Verification items for the finished model (mm, model axes). A direction names the side the tool comes from. Give positions to 0.01 mm unless a question says otherwise; leave off trailing zeros. Loops run counter-clockwise (first coordinate to the right, second up) from the corner with the lowest first, then second, coordinate; pieces in that order, holes last. Notation, with made-up numbers: (-6.75, 66) -> (10.25, 66) arc R21 ccw to (10.25, 74) -> close; hole circle Ø9 at (1.25, 38). An arc over 180 degrees is marked (long way). Use one line per item in the form item = value. Start each with the question number.
from build123d import *

# Parameters (mm, degrees)
BOARD_DEPTH        = 1.68
SKETCH2_R          = 0.2032
SKETCH2_R_2        = 0.4699
SKETCH2_R_3        = 1.5875
SKETCH2_R_4        = 0.4953
PLATED_HOLES_DEPTH = 2.68


with BuildPart() as part:
    # Sketch1 → BOARD (new body)
    with BuildSketch(Plane.XY):
        with BuildLine():
            Line((60, 63), (60, 61))
            ThreePointArc((60, 61), (60.585786438, 59.585786438), (62, 59))
            Line((62, 59), (77.171572667, 59))
            ThreePointArc((77.171572667, 59), (77.936939773, 58.847758994), (78.585786667, 58.414213333))
            Line((78.585786667, 58.414213333), (84.414213333, 52.585786667))
            ThreePointArc((84.414213333, 52.585786667), (85.063060227, 52.152241006), (85.828427333, 52))
            Line((85.828427333, 52), (98, 52))
            ThreePointArc((98, 52), (99.414213562, 52.585786438), (100, 54))
            Line((100, 54), (100, 63))
            ThreePointArc((100, 63), (99.414213562, 64.414213562), (98, 65))
            Line((98, 65), (62, 65))
            ThreePointArc((62, 65), (60.585786438, 64.414213562), (60, 63))
        make_face()
    extrude(amount=BOARD_DEPTH)

    # Sketch2 → PLATED HOLES (cut, through all)
    with BuildSketch(Plane.XY):
        with Locations((67.31, 61.468)):
            Circle(SKETCH2_R)
        with Locations((62.23, 63.5)):
            Circle(SKETCH2_R_2)
        with Locations((64.77, 63.5)):
            Circle(SKETCH2_R_2)
        with Locations((67.31, 63.5)):
            Circle(SKETCH2_R_2)
        with Locations((69.85, 61.1632)):
            Circle(SKETCH2_R)
        with Locations((69.85, 63.5)):
            Circle(SKETCH2_R_2)
        with Locations((82.499999998, 62.000000003)):
            Circle(SKETCH2_R_3)
        with Locations((87.749999989, 55.999999989)):
            Circle(SKETCH2_R_4)
        with Locations((87.749999989, 60.999999996)):
            Circle(SKETCH2_R_4)
        with Locations((94.000000011, 58.499999992)):
            Circle(SKETCH2_R_4)
        with Locations((94.000000011, 55.999999989)):
            Circle(SKETCH2_R_4)
        with Locations((94.000000011, 60.999999996)):
            Circle(SKETCH2_R_4)
    extrude(amount=PLATED_HOLES_DEPTH, mode=Mode.SUBTRACT)


solid = part.part
Item 1: Sectioned sample at D-D, the plane z = 1. State how many separate pieces and enclosed holes the cut face has, and give its area (3 significant figures).
Item 2: Sectioned sample at C-C, the plane x = 81.5. Enter the section's corners in (y, z), and give its area (3 significant figures).
Item 3: Material ranges on line 1 (Y direction, x = 69.85, z = 1); line 2 (Y direction, x = 64.77, z = 0.3); line 3 (X direction, y = 61, z = 1.05), recorded low to high.
Item 4: Tool access check on faces 4 (the flat face through (69, 59, 1)), 5 (the cylindrical face through (94.266, 61.418, 0.828)). Record the directions out of +Z, -Z, +X, -X, +Y, -Y that give a thin tool (end or side, any length) a straight path to the whole face; none if there is none.
Item 5: Sectioned sample at B-B, the plane y = 56. Enter the section's corners in (x, z).
Item 6: Sectioned sample at A-A, the plane x = 94. Enter the section's corners in (y, z), and give its area (3 significant figures).
Item 7: Draft check along X on faces 1 (the flat face through (80, 65, 1)), 2 (the cylindrical face through (60.57, 59.6, 0.83)), 3 (the cylindrical face through (94.266, 58.918, 0.828)). Enter one of: +X half, -X half, draft (parallel to the pull), parting line (faces both ways), or undercut.
Item 8: Gauge pin test, flat ends, axial feed: pin 1 Ø6 at (x, y) = (83.5, 63) entering from +Z; pin 2 Ø0.8 at (x, z) = (70, 0.5) entering from -Y. Record the tip position at first contact, or that the pin passes through.
Outcome:
q1.separate_pieces = 1
q1.enclosed_holes = 12
q1.area = 351 mm^2
q2.outline = (55.5, 0) -> (60.77, 0) -> (60.77, 1.68) -> (55.5, 1.68) -> close; (63.23, 0) -> (65, 0) -> (65, 1.68) -> (63.23, 1.68) -> close
q2.area = 11.8 mm^2
q3.line_1 = 59 to 60.96, 61.37 to 63.03, 63.97 to 65
q3.line_2 = 59 to 63.03, 63.97 to 65
q3.line_3 = 60 to 69.73, 69.97 to 81.27, 83.73 to 87.25, 88.25 to 93.5, 94.5 to 100
q4.face_4 = +Z, -Z, -X, -Y
q4.face_5 = +Z, -Z
q5.outline = (81, 0) -> (87.25, 0) -> (87.25, 1.68) -> (81, 1.68) -> close; (88.25, 0) -> (93.5, 0) -> (93.5, 1.68) -> (88.25, 1.68) -> close; (94.5, 0) -> (100, 0) -> (100, 1.68) -> (94.5, 1.68) -> close
q6.outline = (52, 0) -> (55.5, 0) -> (55.5, 1.68) -> (52, 1.68) -> close; (56.5, 0) -> (58, 0) -> (58, 1.68) -> (56.5, 1.68) -> close; (59, 0) -> (60.5, 0) -> (60.5, 1.68) -> (59, 1.68) -> close; (61.5, 0) -> (65, 0) -> (65, 1.68) -> (61.5, 1.68) -> close
q6.area = 16.8 mm^2
q7.face_1 = draft
q7.face_2 = -X half
q7.face_3 = undercut
q8.pin_1 = 1.68
q8.pin_2 = 59
